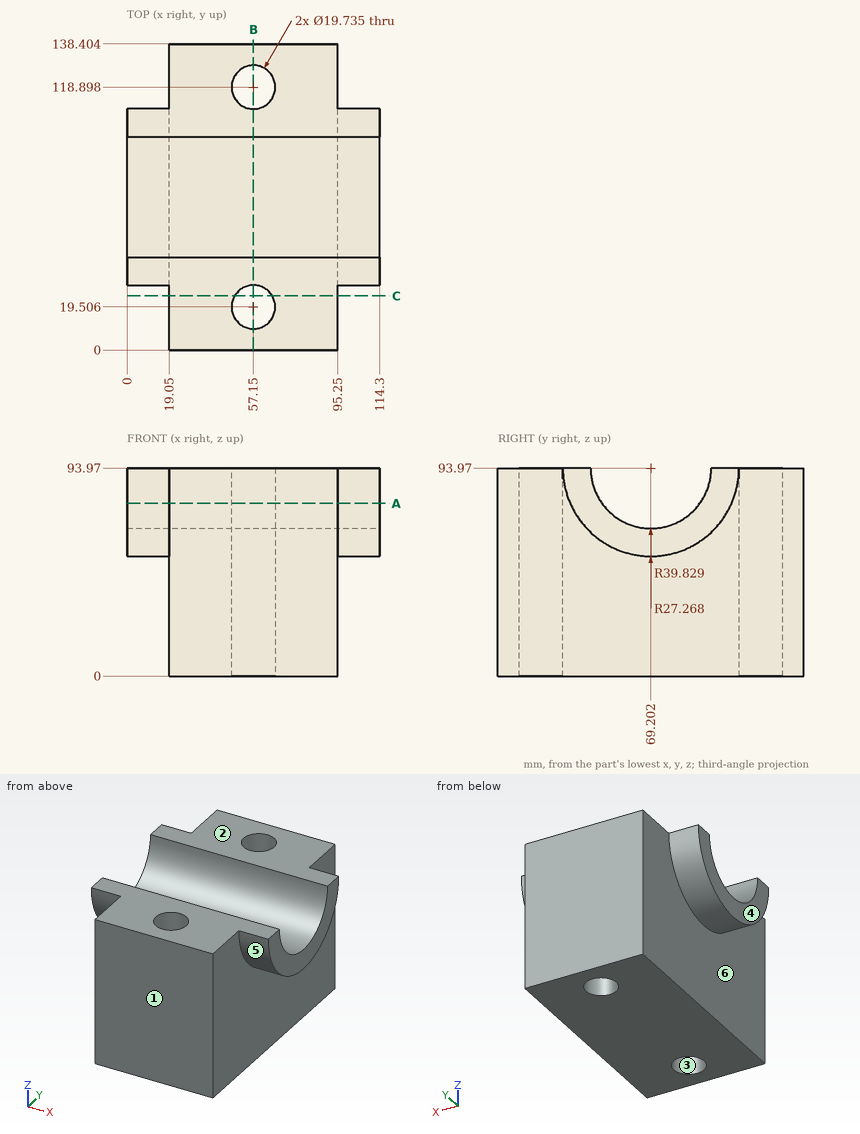
Geometry: see drawing. Coordinates: mm, zero at the bounding-box minimum. A direction names the side the tool comes from. Give positions to 0.01 mm unless a question says otherwise; leave off trailing zeros. Order: outer loops, then holes, each group sorted by start corner. A loop starts at its lowest first (then second) coordinate and runs counter-clockwise, first axis right, second up. Notation, with made-up numbers: (-29, 76) - (0, 76) arc R24 cw to (0, 108) - close; hole circle Ø2 at (-13.5, 26.5). An arc over 180 degrees is marked (long way). Use CSV: the item, a comma, the result in double quotes.
1. Contact query for flat-ended pins moving along their axis: pin 1 (4 mm diameter, centred on y = 65, z = 32, fed in from -X); pin 2 (1 mm diameter, centred on y = 122, z = 50.5, fed in from +X). Output: stop coordinate, or through.
Answers below:
pin 1,"x = 19.05"
pin 2,"x = 95.25"
2. Access query for the marked faces 4, 5 and 6. Directions: +Z, -Z, +X, -X, +Y, -Y. A direction counts if a zero-diameter tool reaches every point of the face in a straight line with its end or side. Return the directions, or none.
Answers below:
face 4,"+Z, -Z, -X, +Y, -Y"
face 5,"-Z, +X"
face 6,"-Z, -X"
3. Material intervals for line 1 along Y through (x, z) = (57, 40) (1 decimal); line 2 along Y through (x, z) = (58, 39) (1 decimal); line 3 along X through (y, z) = (118, 79), sorted ascending. Write a range as from..to.
Answers below:
line 1,"0..9.6, 29.4..109, 128.8..138.4"
line 2,"0..9.7, 29.3..109.1, 128.7..138.4"
line 3,"19.05..47.32, 66.98..95.25"
4. Section query B-B (x = 57.15). Output: boundary loops of the cut face in (y, z) (1 decimal), plus the area to 3 significant figures.
Answers below:
outline,"(0, 0) - (9.6, 0) - (9.6, 94) - (0, 94) - close; (29.4, 0) - (109, 0) - (109, 94) - (96.5, 94) arc R27.3 cw to (41.9, 94) - (29.4, 94) - close; (128.8, 0) - (138.4, 0) - (138.4, 94) - (128.8, 94) - close"
area,"8,130 mm2"
5. Section query A-A (z = 78). Give the number of separate pieces and of enclosed holes in the cut face, plus the area to 3 significant figures.
Answers below:
separate pieces,"2"
enclosed holes,"2"
area,"7,660 mm2"
6. Section query C-C (y = 24.5). Output: boundary loops of the cut face in (x, z), plus the area to 3 significant figures.
Answers below:
outline,"(19.05, 0) - (48.64, 0) - (48.64, 93.97) - (19.05, 93.97) - close; (65.66, 0) - (95.25, 0) - (95.25, 93.97) - (65.66, 93.97) - close"
area,"5,560 mm2"
7. Mould query, pull axis Y, two halves, no side actions, for the marked faces 1, 2 and 3. Classes: +Y half, -Y half, draft (parallel to the pull), parting line (faces both ways), or undercut.
Answers below:
face 1,"-Y half"
face 2,"draft"
face 3,"undercut"
